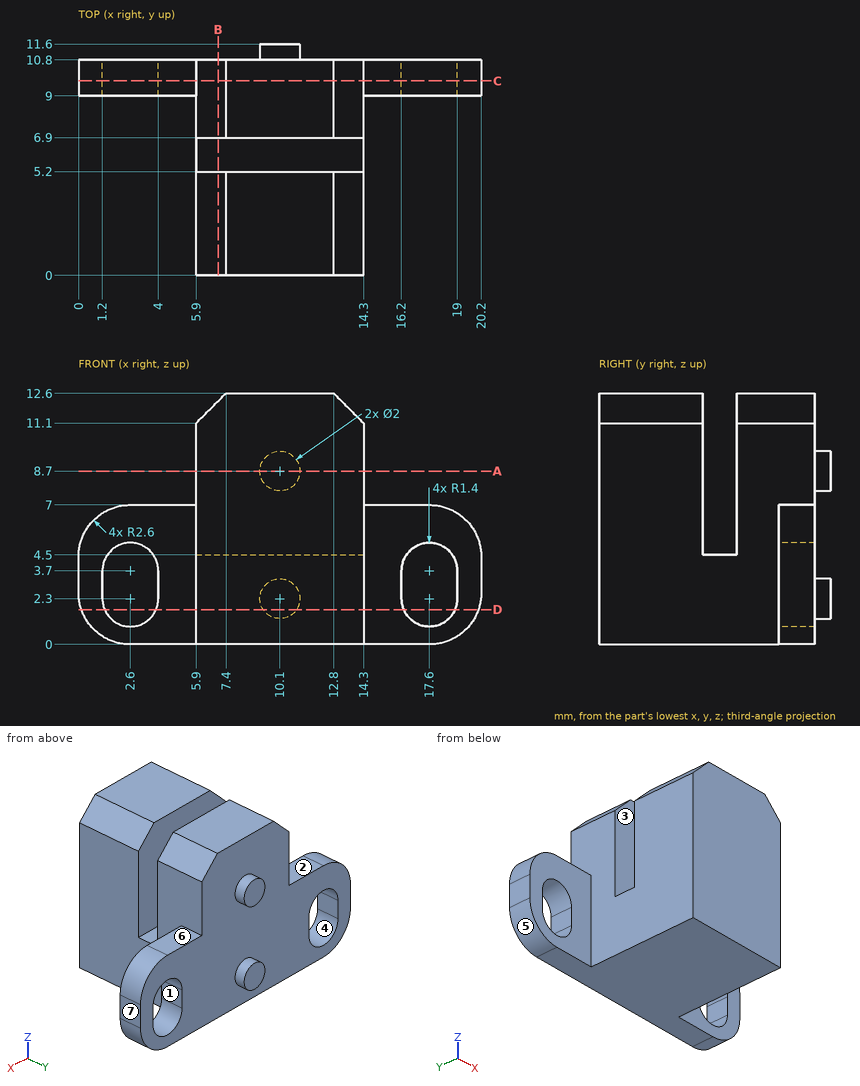
Verification items for this drawing (mm, ordinates from the low corner). A direction names the side the tool comes from. Give positions to 0.01 mm unless a question says otherwise; leave off trailing zeros. Write each loop counter-clockwise with the first axis right and the second up, starting at its lowest first coordinate (ties: lowest second). Pieces come first, ordered by that corner, then holes. Notation, with made-up numbers: (42.5, -14.75) -> (91.5, -14.75) arc R36 cw to (91.5, 19.25) -> close; hole circle Ø3 at (33, 13.25). An arc over 180 degrees is marked (long way). Use one line per item in the form item = value.
Item 1: Depth check by flat-ended pin: pin 1 Ø1.5 at (x, y) = (4.5, 4) entering from +Z; pin 2 Ø0.5 at (x, y) = (15.5, 10.5) entering from +Z; pin 3 Ø1.5 at (x, z) = (15, 8) entering from -Y; pin 4 Ø5.5 at (y, z) = (4, 8) entering from +X. Enter the tip coordinate at first touch or a pass-through.
Results list:
pin_1 = through
pin_2 = 7
pin_3 = 0
pin_4 = 14.3
Item 2: Mould release check, pull along X, two halves, no side actions. Record for the marked faces 4, 5, 6 and 7: released by +X, released by -X, zero draft, split by the parting line, or undercut.
Results list:
face_4 = undercut
face_5 = released by -X
face_6 = zero draft
face_7 = released by +X
Item 3: Access from +Z, -Z, +X, -X, +Y, -Y to the whole of each face (thin tool, end or side, straight path). Record for the marked faces 1, 2 and 3.
Results list:
face_1 = +Y, -Y
face_2 = +Z, -X, +Y, -Y
face_3 = +Z, +X, -X
Item 4: Sectioned sample at D-D on z = 1.75. Enter the section's corners in (x, y).
Results list:
outline = (0.14, 9) -> (1.31, 9) -> (1.31, 10.8) -> (0.14, 10.8) -> close; (3.89, 9) -> (5.9, 9) -> (5.9, 0) -> (14.3, 0) -> (14.3, 9) -> (16.31, 9) -> (16.31, 10.8) -> (10.94, 10.8) -> (10.94, 11.6) -> (9.26, 11.6) -> (9.26, 10.8) -> (3.89, 10.8) -> close; (18.89, 9) -> (20.06, 9) -> (20.06, 10.8) -> (18.89, 10.8) -> close
Item 5: Sectioned sample at B-B on x = 7. Enter the section's corners in (y, z).
Results list:
outline = (0, 0) -> (10.8, 0) -> (10.8, 12.2) -> (6.9, 12.2) -> (6.9, 4.5) -> (5.2, 4.5) -> (5.2, 12.2) -> (0, 12.2) -> close
Item 6: Scan lines: line 1 (X direction, y = 9.5, z = 3); line 2 (Y direction, x = 11.5, z = 7.25); line 3 (X direction, y = 10.75, z = 2). Record each from-to range of solid material in increasing order.
Results list:
line_1 = 0 to 1.2, 4 to 16.2, 19 to 20.2
line_2 = 0 to 5.2, 6.9 to 10.8
line_3 = 0.07 to 1.23, 3.97 to 16.23, 18.97 to 20.13
Item 7: Sectioned sample at C-C on y = 9.75. Enter the section's corners in (x, z).
Results list:
outline = (0, 2.6) arc R2.6 ccw to (2.6, 0) -> (17.6, 0) arc R2.6 ccw to (20.2, 2.6) -> (20.2, 4.4) arc R2.6 ccw to (17.6, 7) -> (14.3, 7) -> (14.3, 11.1) -> (12.8, 12.6) -> (7.4, 12.6) -> (5.9, 11.1) -> (5.9, 7) -> (2.6, 7) arc R2.6 ccw to (0, 4.4) -> close; hole (1.2, 2.3) arc R1.4 ccw to (4, 2.3) -> (4, 3.7) arc R1.4 ccw to (1.2, 3.7) -> close; hole (16.2, 2.3) arc R1.4 ccw to (19, 2.3) -> (19, 3.7) arc R1.4 ccw to (16.2, 3.7) -> close
Item 8: Sectioned sample at A-A on z = 8.7. Enter the section's corners in (x, y), plus the area to 3 significant figures.
Results list:
outline = (5.9, 0) -> (14.3, 0) -> (14.3, 5.2) -> (5.9, 5.2) -> close; (5.9, 6.9) -> (14.3, 6.9) -> (14.3, 10.8) -> (11.1, 10.8) -> (11.1, 11.6) -> (9.1, 11.6) -> (9.1, 10.8) -> (5.9, 10.8) -> close
area = 78.0 mm2
